Check sheet for the modelled part. Datum: model origin and axes. Units: mm. A direction names the side the tool comes from. Coordinates: 2 decimals unless noted, no trailing zeros. Loops run counter-clockwise (first coordinate to the right, second up) from the corner with the lowest first, then second, coordinate; pieces in that order, holes last. Notation, with made-up numbers: M 45.25,77 L 73.25,77 A18 cw 73.25,96 Z; hole C 8,86.5 d4. An arc over 180 degrees is marked long. Return JSON: item names as keys, results as strings.
from build123d import *

# Parameters (mm, degrees)
SKETCH1_W                                      = 196.85
SKETCH1_H                                      = 203.2
BOSS_EXTRUDE1_DEPTH                            = 0.7747
CUT_EXTRUDE7_DEPTH                             = 313.185586086
SKETCH4_W                                      = 196.85
SKETCH4_H                                      = 0.6096
BOSS_EXTRUDE2_DEPTH                            = 12
SKETCH14_W                                     = 196.85
SKETCH14_H                                     = 11.938
BOSS_EXTRUDE3_DEPTH                            = 0.7747
SKETCH13_W                                     = 196.85
SKETCH13_H                                     = 0.6096
CUT_EXTRUDE9_DEPTH                             = 12
CSK_FOR_M3_FLAT_HEAD_MACHINE_SCREW3_AT_2_COUNT = 2
CSK_FOR_M3_FLAT_HEAD_MACHINE_SCREW3_AT_2_PITCH = 150
CSK_FOR_M3_FLAT_HEAD_MACHINE_SCREW3_AT_3_COUNT = 2
CSK_FOR_M3_FLAT_HEAD_MACHINE_SCREW3_AT_3_PITCH = 125
CSK_FOR_M3_FLAT_HEAD_MACHINE_SCREW3_AT_4_COUNT = 2
CSK_FOR_M3_FLAT_HEAD_MACHINE_SCREW3_AT_4_PITCH = 100
CSK_FOR_M3_FLAT_HEAD_MACHINE_SCREW3_AT_5_COUNT = 2
CSK_FOR_M3_FLAT_HEAD_MACHINE_SCREW3_AT_5_PITCH = 75
CSK_FOR_M3_FLAT_HEAD_MACHINE_SCREW3_AT_6_COUNT = 2
CSK_FOR_M3_FLAT_HEAD_MACHINE_SCREW3_AT_6_PITCH = 50
CSK_FOR_M3_FLAT_HEAD_MACHINE_SCREW3_AT_7_COUNT = 2
CSK_FOR_M3_FLAT_HEAD_MACHINE_SCREW3_AT_7_PITCH = 25


with BuildPart() as part:
    # Sketch1 → Boss-Extrude1 (new body)
    with BuildSketch(Plane(origin=(0, 0, 0), x_dir=(1, 0, 0), z_dir=(0, 0, -1))):
        with Locations((-104.775, 135.4)):
            Rectangle(SKETCH1_W, SKETCH1_H)
    extrude(amount=BOSS_EXTRUDE1_DEPTH)

    # Sketch2 → Cut-Extrude7 (cut, through all)
    with BuildSketch(Plane(origin=(0, 0, -0.7747), x_dir=(1, 0, 0), z_dir=(0, 0, -1))):
        with BuildLine():
            Line((-135.221253236, 173.5), (-135.221253236, 148))
            ThreePointArc((-135.221253236, 148), (-141.721253236, 141.5), (-148.221253236, 148))
            Line((-148.221253236, 148), (-148.221253236, 173.5))
            ThreePointArc((-148.221253236, 173.5), (-141.721253236, 180), (-135.221253236, 173.5))
        make_face()
        with BuildLine():
            Line((-62.069253236, 173.5), (-62.069253236, 148))
            ThreePointArc((-62.069253236, 148), (-68.569253236, 141.5), (-75.069253236, 148))
            Line((-75.069253236, 148), (-75.069253236, 173.5))
            ThreePointArc((-75.069253236, 173.5), (-68.569253236, 180), (-62.069253236, 173.5))
        make_face()
    extrude(amount=-CUT_EXTRUDE7_DEPTH, mode=Mode.SUBTRACT)

    # Sketch4 → Boss-Extrude2 (add)
    with BuildSketch(Plane.XY):
        with Locations((-104.775, -34.1048)):
            Rectangle(SKETCH4_W, SKETCH4_H)
    extrude(amount=BOSS_EXTRUDE2_DEPTH)

    # Sketch14 → Boss-Extrude3 (add)
    with BuildSketch(Plane.XY):
        with Locations((-104.775, -53.935004147)):
            Rectangle(SKETCH14_W, SKETCH14_H)
    extrude(amount=-BOSS_EXTRUDE3_DEPTH)

    # Sketch13 → Cut-Extrude9 (cut)
    with BuildSketch(Plane.XY.offset(12)):
        with Locations((-104.775, -34.1048)):
            Rectangle(SKETCH13_W, SKETCH13_H)
    extrude(amount=-CUT_EXTRUDE9_DEPTH, mode=Mode.SUBTRACT)

    # Sketch16 → CSK for M3 Flat Head Machine Screw3 (revolve, cut)
    with BuildSketch(Plane(origin=(-188.645, -72, 0), x_dir=(0, -1, 0), z_dir=(1, 0, 0))):
        Polygon((0, 0), (0, 0.7747), (1.7, 0.7747), (1.7, 2.212), (3.912, 0), align=None)
    csk_for_m3_flat_head_machine_screw3 = revolve(axis=Axis((-188.645, -72, 6.35), (0, 0, -1)), mode=Mode.SUBTRACT)

    # CSK for M3 Flat Head Machine Screw3 at 2: CSK for M3 Flat Head Machine Screw3 ×2
    with Locations(*[(0, -i * CSK_FOR_M3_FLAT_HEAD_MACHINE_SCREW3_AT_2_PITCH, 0) for i in range(1, CSK_FOR_M3_FLAT_HEAD_MACHINE_SCREW3_AT_2_COUNT)]):
        add(csk_for_m3_flat_head_machine_screw3, mode=Mode.SUBTRACT)

    # CSK for M3 Flat Head Machine Screw3 at 3: CSK for M3 Flat Head Machine Screw3 ×2
    with Locations(*[(0, -i * CSK_FOR_M3_FLAT_HEAD_MACHINE_SCREW3_AT_3_PITCH, 0) for i in range(1, CSK_FOR_M3_FLAT_HEAD_MACHINE_SCREW3_AT_3_COUNT)]):
        add(csk_for_m3_flat_head_machine_screw3, mode=Mode.SUBTRACT)

    # CSK for M3 Flat Head Machine Screw3 at 4: CSK for M3 Flat Head Machine Screw3 ×2
    with Locations(*[(0, -i * CSK_FOR_M3_FLAT_HEAD_MACHINE_SCREW3_AT_4_PITCH, 0) for i in range(1, CSK_FOR_M3_FLAT_HEAD_MACHINE_SCREW3_AT_4_COUNT)]):
        add(csk_for_m3_flat_head_machine_screw3, mode=Mode.SUBTRACT)

    # CSK for M3 Flat Head Machine Screw3 at 5: CSK for M3 Flat Head Machine Screw3 ×2
    with Locations(*[(0, -i * CSK_FOR_M3_FLAT_HEAD_MACHINE_SCREW3_AT_5_PITCH, 0) for i in range(1, CSK_FOR_M3_FLAT_HEAD_MACHINE_SCREW3_AT_5_COUNT)]):
        add(csk_for_m3_flat_head_machine_screw3, mode=Mode.SUBTRACT)

    # CSK for M3 Flat Head Machine Screw3 at 6: CSK for M3 Flat Head Machine Screw3 ×2
    with Locations(*[(0, -i * CSK_FOR_M3_FLAT_HEAD_MACHINE_SCREW3_AT_6_PITCH, 0) for i in range(1, CSK_FOR_M3_FLAT_HEAD_MACHINE_SCREW3_AT_6_COUNT)]):
        add(csk_for_m3_flat_head_machine_screw3, mode=Mode.SUBTRACT)

    # CSK for M3 Flat Head Machine Screw3 at 7: CSK for M3 Flat Head Machine Screw3 ×2
    with Locations(*[(0, -i * CSK_FOR_M3_FLAT_HEAD_MACHINE_SCREW3_AT_7_PITCH, 0) for i in range(1, CSK_FOR_M3_FLAT_HEAD_MACHINE_SCREW3_AT_7_COUNT)]):
        add(csk_for_m3_flat_head_machine_screw3, mode=Mode.SUBTRACT)

    # Mirror1: CSK for M3 Flat Head Machine Screw3 across plane
    add(csk_for_m3_flat_head_machine_screw3.mirror(Plane.ZY.offset(104.774999995)), mode=Mode.SUBTRACT)

    # Mirror1 copy 1 sketch → Mirror1 copy 1 (revolve, cut)
    with BuildSketch(Plane(origin=(-20.904999999, -222.000000003, 0), x_dir=(-3.839898042745385e-11, -1.0, 0), z_dir=(-1.0, 3.839898042745385e-11, 0))):
        Polygon((0, 0), (0, -0.7747), (1.7, -0.7747), (1.7, -2.212), (3.912, 0), align=None)
    revolve(axis=Axis((-20.904999999, -222.000000003, 6.35), (0, 0, 1)), mode=Mode.SUBTRACT)

    # Mirror1 copy 2 sketch → Mirror1 copy 2 (revolve, cut)
    with BuildSketch(Plane(origin=(-20.904999998, -197.000000003, 0), x_dir=(-3.839898042745385e-11, -1.0, 0), z_dir=(-1.0, 3.839898042745385e-11, 0))):
        Polygon((0, 0), (0, -0.7747), (1.7, -0.7747), (1.7, -2.212), (3.912, 0), align=None)
    revolve(axis=Axis((-20.904999998, -197.000000003, 6.35), (0, 0, 1)), mode=Mode.SUBTRACT)

    # Mirror1 copy 3 sketch → Mirror1 copy 3 (revolve, cut)
    with BuildSketch(Plane(origin=(-20.904999998, -172.000000003, 0), x_dir=(-3.839898042745385e-11, -1.0, 0), z_dir=(-1.0, 3.839898042745385e-11, 0))):
        Polygon((0, 0), (0, -0.7747), (1.7, -0.7747), (1.7, -2.212), (3.912, 0), align=None)
    revolve(axis=Axis((-20.904999998, -172.000000003, 6.35), (0, 0, 1)), mode=Mode.SUBTRACT)

    # Mirror1 copy 4 sketch → Mirror1 copy 4 (revolve, cut)
    with BuildSketch(Plane(origin=(-20.904999997, -147.000000003, 0), x_dir=(-3.839898042745385e-11, -1.0, 0), z_dir=(-1.0, 3.839898042745385e-11, 0))):
        Polygon((0, 0), (0, -0.7747), (1.7, -0.7747), (1.7, -2.212), (3.912, 0), align=None)
    revolve(axis=Axis((-20.904999997, -147.000000003, 6.35), (0, 0, 1)), mode=Mode.SUBTRACT)

    # Mirror1 copy 5 sketch → Mirror1 copy 5 (revolve, cut)
    with BuildSketch(Plane(origin=(-20.904999996, -122.000000003, 0), x_dir=(-3.839898042745385e-11, -1.0, 0), z_dir=(-1.0, 3.839898042745385e-11, 0))):
        Polygon((0, 0), (0, -0.7747), (1.7, -0.7747), (1.7, -2.212), (3.912, 0), align=None)
    revolve(axis=Axis((-20.904999996, -122.000000003, 6.35), (0, 0, 1)), mode=Mode.SUBTRACT)

    # Mirror1 copy 6 sketch → Mirror1 copy 6 (revolve, cut)
    with BuildSketch(Plane(origin=(-20.904999995, -97.000000003, 0), x_dir=(-3.839898042745385e-11, -1.0, 0), z_dir=(-1.0, 3.839898042745385e-11, 0))):
        Polygon((0, 0), (0, -0.7747), (1.7, -0.7747), (1.7, -2.212), (3.912, 0), align=None)
    revolve(axis=Axis((-20.904999995, -97.000000003, 6.35), (0, 0, 1)), mode=Mode.SUBTRACT)


solid = part.part
1) Section check C-C on y = -97. Record the cut outline in (x, z).
Answers:
{"outline": "M -203.2,-0.77 L -191.78,-0.77 L -192.56,0 L -203.2,0 Z; M -185.51,-0.77 L -24.04,-0.77 L -24.82,0 L -184.73,0 Z; M -17.77,-0.77 L -6.35,-0.77 L -6.35,0 L -16.99,0 Z"}
2) Scan lines: line 1 along X through (y, z) = (-163.5, -0.05); line 2 along X through (y, z) = (-169.5, -0.05); line 3 along Y through (x, z) = (-68.5, -0.6). Record each from-to range of solid material in increasing order. Write a range as [from, to].
Answers:
{"line 1": "[-203.2, -148.22], [-135.22, -75.07], [-62.07, -6.35]", "line 2": "[-203.2, -191.59], [-185.7, -148.22], [-135.22, -75.07], [-62.07, -23.85], [-17.96, -6.35]", "line 3": "[-237, -180], [-141.5, -33.8]"}
3) Section check B-B on z = -0.35. Count the separate pieces of the cut face and the enclosed holes in it, then the cut area to 3 significant figures.
Answers:
{"separate pieces": "1", "enclosed holes": "16", "area": "38,500 mm²"}
4) Set-up check for faces 1 (the face through (-68.7, -180, -0.4)), 2 (the face through (-106, -137, -0.775)): record each of +Z, -Z, +X, -X, +Y, -Y from which the full face is reachable in a straight line by a thin tool's end or side.
Answers:
{"face 1": "+Z, -Z", "face 2": "-Z, +X, -X, +Y, -Y"}
5) Go/stop test with a flat-tipped pin: pin 1 Ø1.5 at (x, y) = (-175.5, -180.5) entering from +Z. Record where the tip stops, or that it passes through.
Answers:
{"pin 1": "z = 0"}
6) Section check A-A on x = -65. Record the cut outline in (y, z), then the cut area to 3 significant figures.
Answers:
{"outline": "M -237,-0.77 L -178.93,-0.77 L -178.93,0 L -237,0 Z; M -142.57,-0.77 L -33.8,-0.77 L -33.8,0 L -142.57,0 Z", "area": "129 mm²"}
7) Draft check along X on faces 3 (the face through (-106, -137, 0)), 4 (the face through (-68.43, -141.5, -0.39)). Enter one of: +X half, -X half, draft (parallel to the pull), parting line (faces both ways), or undercut.
Answers:
{"face 3": "draft", "face 4": "undercut"}
